Autodesk Inventor part; units mm, degrees
ref_plane "YZ Plane" through (0, 0, 0) normal (1, 0, 0) x (0, 1, 0)
ref_plane "XZ Plane" through (0, 0, 0) normal (0, 1, 0) x (-1, 0, 0)
ref_plane "XY Plane" through (0, 0, 0) normal (0, 0, 1) x (1, 0, 0)
sketch "Sketch1" plane through (0, 0, 0) normal (1, 0, 0) x (0, 1, 0)
  circle A0 centre (-4.0069, -0.399) radius 2
  line L0 (-20.007, 88.601) -> (-20.007, 57.351)
  line L1 (-20.007, 57.351) -> (-25.007, 57.351)
  line L2 (-25.007, 88.601) -> (-25.007, 57.351)
  line L3 (-20.007, 88.601) -> (-25.007, 88.601)
  line L4 (-20.007, 31.101) -> (-20.007, -31.899)
  line L5 (-20.007, -31.899) -> (-25.007, -31.899)
  line L6 (-25.007, 31.101) -> (-25.007, -31.899)
  line L7 (-20.007, 31.101) -> (-25.007, 31.101)
  line L8 (-20.007, -58.149) -> (-20.007, -89.399)
  line L9 (-20.007, -89.399) -> (-25.007, -89.399)
  line L10 (-25.007, -58.149) -> (-25.007, -89.399)
  line L11 (-20.007, -58.149) -> (-25.007, -58.149)
  line L12 (19.993, 93.601) -> (19.993, 98.601)
  line L13 (19.993, 98.601) -> (9.9915, 98.601)
  line L14 (9.9915, 93.601) -> (9.9915, 98.601)
  line L15 (-10.0085, 93.601) -> (-10.0085, 98.601)
  line L16 (-25.0077, 98.601) -> (-10.0085, 98.601)
  line L17 (-25.007, 93.601) -> (-25.007, 98.601)
  line L18 (-25.007, 93.601) -> (-33.007, 93.601)
  line L19 (-33.007, 93.601) -> (-33.007, -94.399)
  line L20 (-10.0085, 93.601) -> (9.9915, 93.601)
  line L21 (24.993, -99.399) -> (24.993, -94.399)
  line L22 (9.993, -99.399) -> (24.993, -99.399)
  line L23 (9.993, -99.399) -> (9.993, -94.399)
  line L24 (-10.0077, -94.399) -> (9.993, -94.399)
  line L25 (-10.0077, -99.399) -> (-10.0077, -94.399)
  line L26 (-25.0077, -99.399) -> (-10.0077, -99.399)
  line L27 (-25.0077, -99.399) -> (-25.0077, -94.399)
  line L28 (-33.0079, -94.399) -> (-25.0077, -94.399)
  line L29 (19.993, 93.601) -> (24.993, 93.601)
  line L30 (24.993, -94.399) -> (24.993, -89.399)
  line L31 (19.993, -89.399) -> (24.993, -89.399)
  line L32 (19.993, -89.399) -> (19.993, -58.149)
  line L33 (19.993, -58.149) -> (24.993, -58.149)
  line L34 (24.993, -58.149) -> (24.993, -31.899)
  line L35 (19.993, -31.899) -> (24.993, -31.899)
  line L36 (19.993, -31.899) -> (19.993, 31.101)
  line L37 (19.993, 31.101) -> (24.993, 31.101)
  line L38 (24.993, 31.101) -> (24.993, 57.351)
  line L39 (19.993, 57.351) -> (24.993, 57.351)
  line L40 (19.993, 57.351) -> (19.993, 88.601)
  line L41 (19.993, 88.601) -> (24.993, 88.601)
  line L42 (24.993, 88.601) -> (24.993, 93.601)
  line L43 (24.9931, -99.399) -> (24.9931, -89.399)
  line L44 (24.9931, -89.399) -> (19.9931, -89.399)
  line L45 (19.9931, -89.399) -> (19.9931, -58.149)
  line L46 (19.9931, -58.149) -> (24.9931, -58.149)
  line L47 (24.9931, -58.149) -> (24.9931, -31.899)
  line L48 (24.9931, -31.899) -> (19.9931, -31.899)
  line L49 (19.9931, -31.899) -> (19.9931, 31.101)
  line L50 (19.9931, 31.101) -> (24.9931, 31.101)
  line L51 (24.9931, 31.101) -> (24.9931, 57.351)
  line L52 (24.9931, 57.351) -> (19.9931, 57.351)
  line L53 (19.9931, 57.351) -> (19.9931, 88.601)
  line L54 (19.9931, 88.601) -> (24.9931, 88.601)
  line L55 (24.9931, 88.601) -> (24.9931, 93.601)
  line L56 (-33.0069, 93.601) -> (-33.0069, 33.601)
  circle A1 centre (-4.0069, -0.399) radius 2
  line L57 (-20.007, -89.399) -> (-25.007, -89.399)
  line L58 (-25.007, -89.399) -> (-25.007, -58.149)
  line L59 (-25.007, -58.149) -> (-20.007, -58.149)
  line L60 (-20.007, -58.149) -> (-20.007, -89.399)
  line L61 (-20.007, -31.899) -> (-25.007, -31.899)
  line L62 (-25.007, -31.899) -> (-25.007, 31.101)
  line L63 (-25.007, 31.101) -> (-20.007, 31.101)
  line L64 (-20.007, 31.101) -> (-20.007, -31.899)
  line L65 (-20.007, 57.351) -> (-25.007, 57.351)
  line L66 (-25.007, 57.351) -> (-25.007, 88.601)
  line L67 (-25.007, 88.601) -> (-20.007, 88.601)
  line L68 (-20.007, 88.601) -> (-20.007, 57.351)
  dimension "d24" = 4
  dimension "d25" = 8
  dimension "d27" = 198
  dimension "d30" = 5
  dimension "d31" = 188
  dimension "d32" = 188
  dimension "d33" = 58
  dimension "d35" = 5
  dimension "d36" = 24
extrude "Extrusion1" add sketch "Sketch1" along normal blind 5
properties part number "case top sides" material "ABS Plastic"
CAD build for the part. Positions are in the model's coordinates, mm. A direction names the side the tool comes from. Round coordinates to 2 decimals unless told otherwise and drop trailing zeros. Order: outer loops, then holes, each group sorted by start corner. A loop starts at its lowest first (then second) coordinate and runs counter-clockwise, first axis right, second up. Notation, with made-up numbers: (-38.75, 39) -> (16.25, 39) arc R37 cw to (16.25, 78) -> close; hole circle Ø6 at (25.5, -13.75). An arc over 180 degrees is marked (long way). Write item = value, one per line.
(1) Pull direction Z, two halves, no side cores. Call faces 1 (the flat face through (2, 24.993, 44)), 2 (the flat face through (2, -18, 98.601)), 3 (the flat face through (2, -25.007, 73)): +Z half, -Z half, draft (parallel to the pull), parting line (faces both ways), or undercut.
Answers follow:
face_1 = draft
face_2 = +Z half
face_3 = undercut
(2) Flat gauge pins, fed straight in: P1, Ø1.5, axis at x = 3, z = -0.5, coming from the +Y side; P2, Ø1.5, axis at x = 1.5, y = -0.5, coming from the -Z side; P3, Ø1.5, axis at x = 2.5, y = 21, coming from the +Z side. Where does each tip first touch, or does it go through?
Answers follow:
P1 = 19.99
P2 = -94.4
P3 = 93.6
(3) Cut at A-A (z = -22). Write the cut outline in (x, y).
Answers follow:
outline = (0, -33.01) -> (5, -33.01) -> (5, -25.01) -> (0, -25.01) -> close; (0, -20.01) -> (5, -20.01) -> (5, 19.99) -> (0, 19.99) -> close
(4) Cut at C-C (x = 2.6). State how many separate pieces and enclosed holes the cut face has, plus the area to 3 significant figures.
Answers follow:
separate_pieces = 1
enclosed_holes = 4
area = 9,910 mm²
(5) Cut at B-B (y = 3). Write the cut outline in (x, z), plus the area to 3 significant figures.
Answers follow:
outline = (0, -94.4) -> (5, -94.4) -> (5, 93.6) -> (0, 93.6) -> close
area = 940 mm²
(6) 3-axis set-ups, long thin cutter, end or side, ignore diameter. For faces 4 (the flat face through (2, 22, 88.601)), 5 (the flat face through (2, -22, -31.899)), 6 (the flat face through (2, -10.008, 96)): which of +Z, -Z, +X, -X, +Y, -Y reach the whole face in a straight line?
Answers follow:
face_4 = +X, -X, +Y
face_5 = +X, -X
face_6 = +Z, +X, -X
(7) Drill centre lines: L1, parallel to Z at x = 3.05, y = -21; L2, parallel to Y at x = 4.4, z = -76; L3, parallel to Z at x = 2.3, y = -7. Where is each one in solid material? Low to high.
Answers follow:
L1 = -99.4 to -89.4, -58.15 to -31.9, 31.1 to 57.35, 88.6 to 98.6
L2 = -33.01 to -25.01, -20.01 to 19.99
L3 = -94.4 to 93.6
